Read the model definition and answer for the solid it produces. Units are mm, in the model's axes. Face numbers are marked on the shaded views. Coordinates: 2 decimals unless noted, no trailing zeros. Order: outer loops, then holes, each group sorted by start corner. A loop starts at its lowest first (then second) coordinate and runs counter-clockwise, first axis right, second up.
```python
from build123d import *

# Parameters (mm, degrees)
SKETCH1_W           = 362
SKETCH1_H           = 357
BOSS_EXTRUDE1_DEPTH = 158
SKETCH2_R           = 62.877116211
CUT_EXTRUDE1_DEPTH  = 60
REVOLVE1_ANGLE      = 180
REVOLVE2_ANGLE      = 180


with BuildPart() as part:
    # Sketch1 → Boss-Extrude1 (new body)
    with BuildSketch(Plane(origin=(0, 0, 0), x_dir=(1, 0, 0), z_dir=(0, 1, 0))):
        Rectangle(SKETCH1_W, SKETCH1_H)
    extrude(amount=BOSS_EXTRUDE1_DEPTH)

    # Sketch2 → Cut-Extrude1 (cut)
    with BuildSketch(Plane(origin=(181, 0, 0), x_dir=(0, 0, -1), z_dir=(1, 0, 0))):
        with Locations((-79.77402599, 79)):
            Circle(SKETCH2_R)
        with Locations((79.77402599, 79)):
            Circle(SKETCH2_R)
    extrude(amount=-CUT_EXTRUDE1_DEPTH, mode=Mode.SUBTRACT)

    # Sketch3 → Revolve1 (revolve)
    with BuildSketch(Plane(origin=(121, 0, 0), x_dir=(0, 0, -1), z_dir=(1, 0, 0))):
        with BuildLine():
            Line((-79.77402599, 141.877116211), (-79.77402599, 16.122883789))
            ThreePointArc((-79.77402599, 16.122883789), (-142.651142201, 79), (-79.77402599, 141.877116211))
        make_face()
    revolve(axis=Axis((121, 141.877116211, 79.77402599), (0, 1, 0)), revolution_arc=REVOLVE1_ANGLE)

    # Sketch4 → Revolve2 (revolve)
    with BuildSketch(Plane(origin=(121, 0, 0), x_dir=(0, 0, -1), z_dir=(1, 0, 0))):
        with BuildLine():
            Line((79.77402599, 141.877116211), (79.77402599, 16.122883789))
            ThreePointArc((79.77402599, 16.122883789), (16.896909779, 79), (79.77402599, 141.877116211))
        make_face()
    revolve(axis=Axis((121, 141.877116211, -79.77402599), (0, 1, 0)), revolution_arc=REVOLVE2_ANGLE)


solid = part.part
```
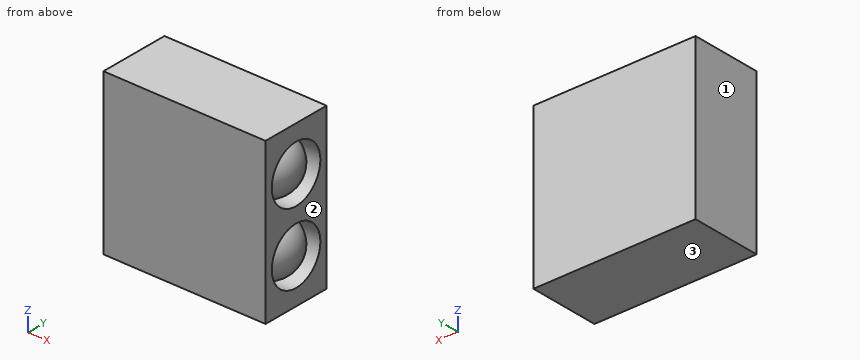
1) A cutting plane is placed at A-A, the plane x = 140.5. Determine the outline of the cut face in (y, z).
A:
outline: (0, -178.5) - (158, -178.5) - (158, 178.5) - (0, 178.5) - close; circle Ø119.55 at (79, -79.77); circle Ø119.55 at (79, 79.77); hole circle Ø125.75 at (79, -79.77); hole circle Ø125.75 at (79, 79.77)
2) A cutting plane is placed at D-D, the plane y = 101. Determine the outline of the cut face in (x, z), and give its area (3 significant figures).
A:
outline: (-181, -178.5) - (181, -178.5) - (181, -138.68) - (121, -138.68) arc R58.9 ccw to (121, -20.87) - (181, -20.87) - (181, 20.87) - (121, 20.87) arc R58.9 ccw to (121, 138.68) - (181, 138.68) - (181, 178.5) - (-181, 178.5) - close
area: 126,000 mm2
3) Determine the mould class of the marked faces 1, 2 and 3 for opening direction X: pulls with the +X half, pulls with the -X half, needs draft (parallel to the pull), parting line crosses it, or undercut.
A:
face 1: pulls with the -X half
face 2: pulls with the +X half
face 3: needs draft
4) A flat-ended cylindrical pin translates along its axis: pin 1 Ø4 at (x, z) = (41, -85.5) entering from -Y. Find the tip coordinate at first contact, or state that the pin passes through.
A:
pin 1: stops at y = 0
5) A cutting plane is placed at B-B, the plane y = 38.5. Determine the outline of the cut face in (x, z), and give its area (3 significant figures).
A:
outline: (-181, -178.5) - (181, -178.5) - (181, -127.87) - (121, -127.87) arc R48.1 ccw to (121, -31.68) - (181, -31.68) - (181, 31.68) - (121, 31.68) arc R48.1 ccw to (121, 127.87) - (181, 127.87) - (181, 178.5) - (-181, 178.5) - close
area: 125,000 mm2
6) Straight lines are drawn through the part: line 1 (Z direction, x = 165, y = 79); line 2 (Y direction, x = 129.5, z = 70.5); line 3 (Z direction, x = 163, y = 79). For each, find the intervals that lie inside material, in ascending order.
A:
line 1: z = -178.5 to -142.65, -124.69 to -34.86, -16.9 to 16.9, 34.86 to 124.69, 142.65 to 178.5
line 2: y = 0 to 16.81, 17.39 to 140.61, 141.19 to 158
line 3: z = -178.5 to -142.65, -126.57 to -32.98, -16.9 to 16.9, 32.98 to 126.57, 142.65 to 178.5
7) A cutting plane is placed at C-C, the plane z = -48. Determine the outline of the cut face in (x, y).
A:
outline: (-181, 0) - (181, 0) - (181, 24.74) - (121, 24.74) arc R54.26 ccw to (121, 133.26) - (181, 133.26) - (181, 158) - (-181, 158) - close
